Could you check a few things on this model? Use its own coordinates, in mm. Give positions to 0.01 mm unless a question says otherwise; leave off trailing zeros. Order: outer loops, then holes, each group sorted by start corner. A loop starts at its lowest first (then second) coordinate and runs counter-clockwise, first axis right, second up. Notation, with made-up numbers: M 57,57 L 99,57 A30 ccw 99,79 Z; hole C 17.5,22 d9. An arc over 180 degrees is marked long. Use a Markdown table: item, result. Add a question column.
Item 1: Suppose I cut it at A-A on x = 0. Write out the boundary of the cut face in (y, z), plus the area to 3 significant figures.
Item 2: Suppose I cut it at D-D on z = 6.5. Write out the boundary of the cut face in (x, y).
Item 3: Suppose I cut it at C-C on y = -0.6. Write out the boundary of the cut face in (x, z), plus the area to 3 significant figures.
Item 4: Suppose I cut it at B-B on z = 9.5. Write out the boundary of the cut face in (x, y).
Item 5: If I drill on L1, parallel to Z at x = 0, y = -1.7; L2, parallel to X at y = -0.55, z = 9.25; L3, parallel to X at y = -0.35, z = 9.5, over which ranges is the centre line in solid material (lowest first)? Write a range as from..to.
Item 6: I'm going to push flat-ended pins straight in: pin 1 Ø3 at (x, z) = (0, 8.45) entering from -Y; pin 2 Ø1.5 at (x, y) = (-1.5, -1.5) entering from +Z. Where does each tip first touch, or does it pass through?
Item 7: If we mould it in two halves opening along X, with no side actions, what happens to faces 1 (the face through (-0.163, -1.232, 9.693)), 2 (the face through (-0.786, -1.232, 11.607)), 3 (the face through (5.058, -1.232, 6.218))? For each: released by +X, released by -X, zero draft, split by the parting line, or undercut.
from build123d import *

# Parameters (mm, degrees)
F0_R     = 1.25
F1_DEPTH = 2.5


with BuildPart() as f1:
    # F0 (on Front) → F1 (new body)
    with BuildSketch(Plane.XZ):
        with BuildLine():
            ThreePointArc((-3.249998, 8.457035), (-0.001773, 5.203488), (3.25, 8.453488))
            ThreePointArc((3.25, 8.453488), (3.138074, 9.299061), (2.810004, 10.086393))
            ThreePointArc((2.810004, 10.086393), (-0.843861, 11.592022), (-3.249998, 8.457035))
        make_face()
        with Locations((0, 8.453488)):
            Circle(F0_R, mode=Mode.SUBTRACT)
        with BuildLine():
            ThreePointArc((2.810004, 10.086393), (3.138074, 9.299061), (3.25, 8.453488))
            ThreePointArc((3.25, 8.453488), (-0.001773, 5.203488), (-3.249998, 8.457035))
            Line((-3.249998, 8.457035), (-3.256546, 2.457038))
            Line((-3.256546, 2.457038), (7.243454, 2.457038))
            Line((7.243454, 2.457038), (2.810004, 10.086393))
        make_face()
    extrude(amount=F1_DEPTH)


solid = f1.part
Findings below:
| question | item | result |
|---|---|---|
| 1 | outline | M -2.5,2.46 L 0,2.46 L 0,7.2 L -2.5,7.2 Z; M -2.5,9.7 L 0,9.7 L 0,11.7 L -2.5,11.7 Z |
| 1 | area | 16.9 mm^2 |
| 2 | outline | M -3.25,-2.5 L 4.89,-2.5 L 4.89,0 L -3.25,0 Z |
| 3 | outline | M -3.26,2.46 L 7.24,2.46 L 2.81,10.09 A3.25 ccw -3.25,8.46 Z; hole C 0,8.45 d2.5 |
| 3 | area | 64.5 mm^2 |
| 4 | outline | M -3.08,-2.5 L -0.68,-2.5 L -0.68,0 L -3.08,0 Z; M 0.68,-2.5 L 3.15,-2.5 L 3.15,0 L 0.68,0 Z |
| 5 | L1 | z = 2.46..7.2, 9.7..11.7 |
| 5 | L2 | x = -3.15..-0.96, 0.96..3.3 |
| 5 | L3 | x = -3.08..-0.68, 0.68..3.15 |
| 6 | pin 1 | stops at y = -2.5 |
| 6 | pin 2 | stops at z = 11.62 |
| 7 | face 1 | undercut |
| 7 | face 2 | split by the parting line |
| 7 | face 3 | released by +X |
